The model under review builds one solid part; all positions refer to its coordinate system, in mm. Round coordinates to 2 decimals unless told otherwise and drop trailing zeros. Order: outer loops, then holes, each group sorted by start corner. A loop starts at its lowest first (then second) coordinate and runs counter-clockwise, first axis right, second up. Notation, with made-up numbers: (62.25, 48) -> (107.25, 48) arc R27 ccw to (107.25, 86) -> close; hole circle Ø11 at (69, 36). An arc over 180 degrees is marked (long way). Put each result on its own line as item: value. Start each with the question number.
Autodesk Inventor part; units mm, degrees
ref_plane "YZ Plane" through (0, 0, 0) normal (1, 0, 0) x (0, 1, 0)
ref_plane "XZ Plane" through (0, 0, 0) normal (0, 1, 0) x (-1, 0, 0)
ref_plane "XY Plane" through (0, 0, 0) normal (0, 0, 1) x (1, 0, 0)
sketch "Sketch1" plane through (0, 0, 0) normal (0, 0, 1) x (1, 0, 0)
  circle A0 centre (0, 0) radius 10
  line L0 (50, -20) -> (50, 20)
  arc A1 (49.8462, 20.7692) -> (49.8462, -20.7692) centre (0, 0) ccw
  arc A2 (50, 20) -> (49.8462, 20.7692) centre (48, 20) ccw
  arc A3 (49.8462, -20.7692) -> (50, -20) centre (48, -20) ccw
  point P0 (50, -20.3961)
  point P1 (50, 20.3961)
  dimension "d1" = 20
  dimension "d12" = 50
  dimension "d14" = 54
extrude "Extrusion3" add sketch "Sketch1" along normal blind 3
properties part number "EndCap 108 Cover"
Q1. Take a section at C-C on z = 2. Give the boundary of the cut face in (x, y), and give its area (3 significant figures).
Q2. Take a section at D-D on y = 39.5. Give the boundary of the cut face in (x, z), and give its area (3 significant figures).
Q3. Clearance check with flat-ended pins moving along their axes: pin 1 Ø18 at (x, y) = (0, 0) entering from +Z; pin 2 Ø1 at (x, z) = (-6, 2) entering from +Y; pin 3 Ø1.5 at (y, z) = (-15, 2.5) entering from -X; pin 4 Ø5 at (x, y) = (25.5, 35) entering from -Z. State where each tip first meets the part, or that it passes through.
Q4. Wall thickness on probe 1 along Y at (x, z) = (0, 0.8); probe 2 along X at (y, z) = (4.5, 0.7); probe 3 along X at (y, z) = (41, 1.75): over which ranges is each line inside the solid? List them lowest first. Write a range as [from, to].
Q5. Take a section at A-A on x = 0. Give the boundary of the cut face in (y, z).
Q6. Draft analysis for pull direction X (two halves, no side actions). For faces 1 (the face through (-3, -11, 0)), 2 (the face through (50, 0, 1)), 3 (the face through (-2.17, 9.76, 1.48)), state which applies: +X half, -X half, draft (parallel to the pull), parting line (faces both ways), or undercut.
Q7. Take a section at B-B on y = 0. Give the boundary of the cut face in (x, z).
Calculated:
1. outline: (49.85, -20.77) arc R2 ccw to (50, -20) -> (50, 20) arc R2 ccw to (49.85, 20.77) arc R54 ccw (long way) to start; hole circle Ø20 at (0, 0)
1. area: 8,740 mm²
2. outline: (-36.82, 0) -> (36.82, 0) -> (36.82, 3) -> (-36.82, 3) -> close
2. area: 221 mm²
3. pin 1: passes through
3. pin 2: stops at y = 53.72
3. pin 3: stops at x = -52.09
3. pin 4: stops at z = 0
4. probe 1: y = [-54, -10], [10, 54]
4. probe 2: x = [-53.81, -8.93], [8.93, 50]
4. probe 3: x = [-35.14, 35.14]
5. outline: (-54, 0) -> (-10, 0) -> (-10, 3) -> (-54, 3) -> close; (10, 0) -> (54, 0) -> (54, 3) -> (10, 3) -> close
6. face 1: draft
6. face 2: +X half
6. face 3: undercut
7. outline: (-54, 0) -> (-10, 0) -> (-10, 3) -> (-54, 3) -> close; (10, 0) -> (50, 0) -> (50, 3) -> (10, 3) -> close
